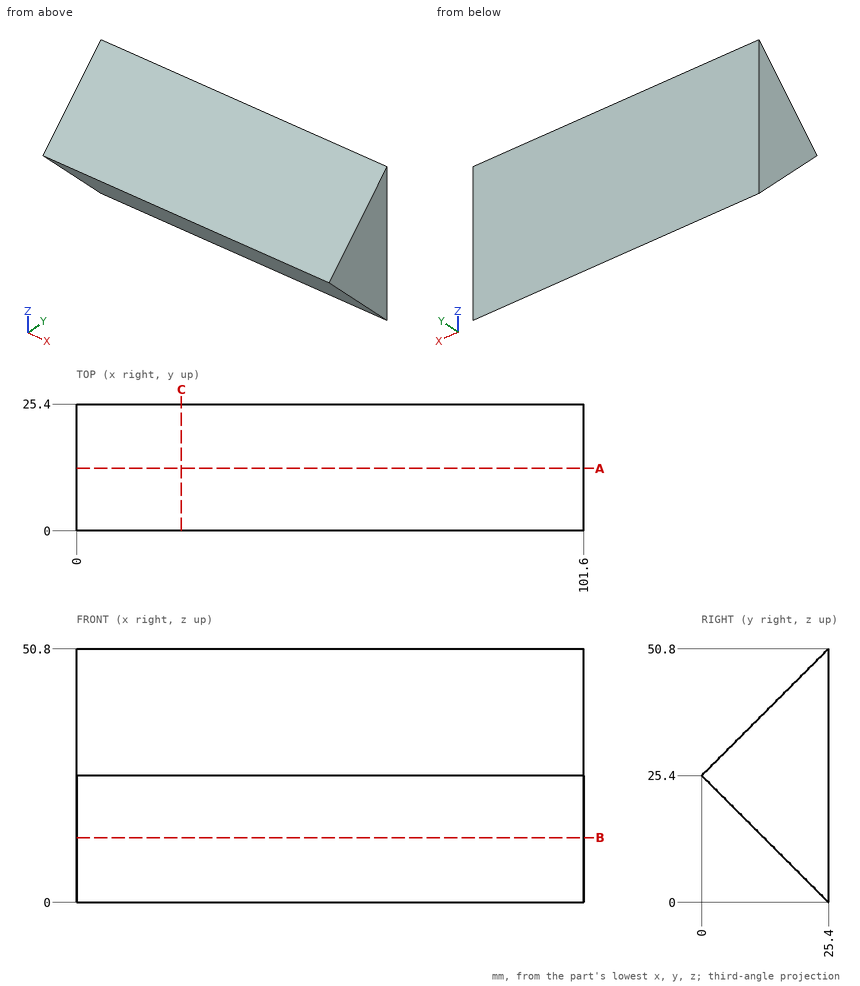
Job drawing, mm, ordinate dimensions from the low corner. One solid piece. Give positions to 0.01 mm unless a question says otherwise; leave off trailing zeros. Loops run counter-clockwise (first coordinate to the right, second up) from the corner with the lowest first, then second, coordinate; pieces in that order, holes last. Notation, with made-up numbers: (32, -33.5) - (70, -33.5) arc R4 ccw to (70, -26.5) - close; hole circle Ø1 at (27, 85.25). An arc over 180 degrees is marked (long way). Use one line per item in the form item = value.
(1) Drill centre lines: L1, parallel to Y at x = 90.5, z = 41.5; L2, parallel to Y at x = 31, z = 5.5; L3, parallel to Z at x = 56, y = 22. Where is each one in solid material? Low to high.
Determined:
L1 = 16.1 to 25.4
L2 = 19.9 to 25.4
L3 = 3.4 to 47.4
(2) Cut at B-B (z = 13). Give the cut face in (x, y), then the cut area to 3 significant figures.
Determined:
outline = (0, 12.4) - (101.6, 12.4) - (101.6, 25.4) - (0, 25.4) - close
area = 1,320 mm^2
(3) Cut at C-C (x = 21). Give the cut face in (y, z), then the cut area to 3 significant figures.
Determined:
outline = (0, 25.4) - (25.4, 0) - (25.4, 50.8) - close
area = 645 mm^2
(4) Drop flat-ended pins along their axis: P1, Ø6, axis at x = 39.5, z = 32, coming from the -Y side; P2, Ø5, axis at x = 51, y = 15.5, coming from the -Z side; P3, Ø10, axis at y = 7.5, z = 15.5, coming from the +X side. Give the stop position or say it passes through.
Determined:
P1 = 3.6
P2 = 7.4
P3 = 101.6
(5) Cut at A-A (y = 12.5). Give the cut face in (x, z), then the cut area to 3 significant figures.
Determined:
outline = (0, 12.9) - (101.6, 12.9) - (101.6, 37.9) - (0, 37.9) - close
area = 2,540 mm^2
